Source: CAD feature listing. Evaluate the final solid. Frame: model axes, mm. Face numbers are marked on the shaded views. A direction names the side the tool comes from. Give positions to 0.01 mm unless a question says otherwise; leave off trailing zeros. Loops run counter-clockwise (first coordinate to the right, second up) from the corner with the lowest first, then second, coordinate; pieces in that order, holes last.
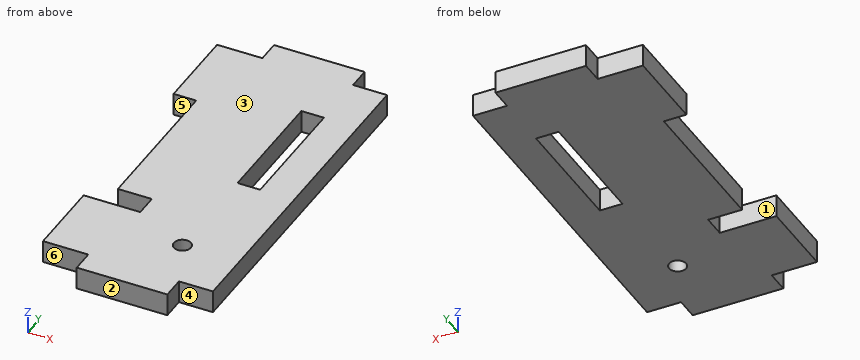
Autodesk Inventor part; units mm, degrees
ref_plane "YZ Plane" through (0, 0, 0) normal (1, 0, 0) x (0, 1, 0)
ref_plane "XZ Plane" through (0, 0, 0) normal (0, 1, 0) x (-1, 0, 0)
ref_plane "XY Plane" through (0, 0, 0) normal (0, 0, 1) x (1, 0, 0)
sketch "Эскиз1" plane through (0, 0, 0) normal (0, 0, 1) x (1, 0, 0)
  line L0 (-12, -16) -> (-12, -30)
  line L1 (-12, -30) -> (-4, -30)
  line L2 (-4, -34) -> (12, -34)
  line L3 (12, -34) -> (12, -2)
  line L4 (-8, 0) -> (8, 0)
  line L5 (-4, -30) -> (-4, -34)
  line L6 (-12, 30) -> (-4, 30)
  line L7 (-4, 34) -> (12, 34)
  line L8 (-4, 30) -> (-4, 34)
  line L9 (12, 34) -> (12, 20)
  line L10 (12, 20) -> (8, 20)
  line L11 (8, 20) -> (8, -2)
  line L12 (8, -2) -> (12, -2)
  line L13 (-8, -12) -> (-8, 15)
  line L14 (-8, 15) -> (-12, 15)
  line L15 (-12, 15) -> (-12, 30)
  line L16 (-8, -12) -> (-2, -12)
  line L17 (-2, -12) -> (-2, -16)
  line L18 (-2, -16) -> (-12, -16)
  point P0 (0, 0)
  point P1 (0, 0)
  dimension "d0" = 16
  dimension "d1" = 8
  dimension "d12" = 60
  dimension "d17" = 22
  dimension "d18" = 14
  dimension "d19" = 27
  dimension "d20" = 10
  dimension "d21" = 4
  dimension "d22" = 15
extrude "Выдавливание1" add sketch "Эскиз1" along normal blind 4
sketch "Эскиз2" plane through (0, 0, 4) normal (0, 0, 1) x (1, 0, 0)
  circle A0 centre (8, -21) radius 1.5
  line L0 (-12, -16) -> (-12, -30)
  line L1 (-12, -30) -> (-4, -30)
  point P0 (0, 0)
  dimension "d23" = 20
  dimension "d24" = 9
  dimension "d25" = 3
extrude "Выдавливание2" cut sketch "Эскиз2" against normal through all
sketch "Эскиз3" plane through (0, 0, 4) normal (0, 0, 1) x (1, 0, 0)
  line L0 (12, 20) -> (12, 34)
  line L1 (12, 30) -> (18, 30)
  line L2 (18, 30) -> (18, -30)
  line L3 (18, -30) -> (12, -30)
  line L4 (12, -30) -> (12, 30)
  point P0 (0, 0)
  point P1 (-4, 30)
  point P2 (-4, -30)
  dimension "d28" = 6
extrude "Выдавливание3" add sketch "Эскиз3" against normal up to surface (4 mm away)
properties part number "batTop" material "Дерево (береза)"
(1) Section C-C, the plane z = 3.05. Return the cut outline in (x, y).
A:
outline: (-12, -30) - (-4, -30) - (-4, -34) - (12, -34) - (12, -30) - (18, -30) - (18, 30) - (12, 30) - (12, 34) - (-4, 34) - (-4, 30) - (-12, 30) - (-12, 15) - (-8, 15) - (-8, -12) - (-2, -12) - (-2, -16) - (-12, -16) - close; hole circle Ø3 at (8, -21); hole (8, -2) - (12, -2) - (12, 20) - (8, 20) - close
(2) First-contact query: pin 1 (2 mm diameter, centred on x = -10.5, z = 3, fed in from -Y); pin 2 (1.2 mm diameter, centred on x = 14.5, z = 2.5, fed in from +Y); pin 3 (1.2 mm diameter, centred on y = 8, z = 1.5, fed in from -X). Flat tips, straight axial feed; report the tip coordinate or a pass-through.
A:
pin 1: stops at y = -30
pin 2: stops at y = 30
pin 3: stops at x = -8
(3) Section D-D, the plane x = 13.5. Return the cut outline in (y, z), then the cut area to 3 significant figures.
A:
outline: (-30, 0) - (30, 0) - (30, 4) - (-30, 4) - close
area: 240 mm2
(4) Ray query, line 1 along Y through (x, z) = (-3.25, 2.5); line 2 along Y through (x, z) = (10, 3.6); line 3 along X through (y, z) = (-30.5, 3.05). Return the intervals inside material, ascending.
A:
line 1: y = -34 to -16, -12 to 34
line 2: y = -34 to -2, 20 to 34
line 3: x = -4 to 12
(5) Section A-A, the plane x = -3. Return the cut outline in (y, z).
A:
outline: (-34, 0) - (-16, 0) - (-16, 4) - (-34, 4) - close; (-12, 0) - (34, 0) - (34, 4) - (-12, 4) - close
(6) Reachability of the marked faces 4, 5 and 6 from +Z, -Z, +X, -X, +Y, -Y: full face, straight path, thin tool, end or side. Return the list, or none.
A:
face 4: +Z, -Z, +X, -Y
face 5: +Z, -Z, -X
face 6: +Z, -Z, -X, -Y
(7) Section B-B, the plane y = -21. Return the cut outline in (x, z).
A:
outline: (-12, 0) - (6.5, 0) - (6.5, 4) - (-12, 4) - close; (9.5, 0) - (18, 0) - (18, 4) - (9.5, 4) - close
(8) Mould query, pull axis Y, two halves, no side actions, for the marked faces 1, 2 and 3. Classes: pulls with the +Y half, pulls with the -Y half, needs draft (parallel to the pull), parting line crosses it, or undercut.
A:
face 1: undercut
face 2: pulls with the -Y half
face 3: needs draft
